Design review of the part built by this model. Coordinates are the model's own, in mm. Round coordinates to 2 decimals unless told otherwise and drop trailing zeros. Loops run counter-clockwise (first coordinate to the right, second up) from the corner with the lowest first, then second, coordinate; pieces in that order, holes last. Notation, with made-up numbers: (46, 80.5) - (68, 80.5) arc R35 cw to (68, 118.5) - close; hole circle Ø3 at (-0.75, 52). An arc over 180 degrees is marked (long way). Return JSON: item names as keys, results as strings. Group by question number.
(1) We need section B-B, the plane x = 0. Write out the cut boundary in (y, z) (3 decimals).
(2) We need section D-D, the plane y = -28. Write out the cut boundary in (x, z).
(3) The part is to be moulded in two halves that separate along Y. For faces 1 (the cylindrical face through (95.38, 30.04, -0.01)), 2 (the cylindrical face through (16.5, -12.3, 0)), 3 (the cylindrical face through (-21.24, 10.87, -0.01)), 4 (the flat face through (21, 1, -0.9)), say which applies: pulls with the +Y half, pulls with the -Y half, needs draft (parallel to the pull), parting line crosses it, or undercut.
(4) We need section C-C, the plane y = 0. Write out the cut boundary in (x, z) (3 decimals).
(5) Clearance check with flat-ended pins moving along their axes: pin 1 (1 mm diameter, centred on x = 70, z = -0.5, fed in from +Y); pin 2 (7 mm diameter, centred on x = 18.62, y = 10.75, fed in from +Z). State where each tip first meets the part, or that it passes through.
(6) Wall thickness on L1, parallel to Y at x = 0, z = 0.25 (3 decimals); L2, parallel to X at y = -23, z = 0.5; L3, parallel to Y at x = 6, z = -0.1: over which ranges is each line inside the solid? List them lowest first. Write a range as [from, to].
(7) We need section A-A, the plane z = 0.55. Write out the cut boundary in (x, y) (3 decimals), and give its area (3 significant figures).
from build123d import *

# Parameters (mm, degrees)
BOSS_EXTRUDE1_DEPTH      = 0.9
BOSS_EXTRUDE1_DEPTH_BACK = 0.9
SKETCH1_R                = 100
SKETCH1_R_2              = 16.625
SKETCH1_R_3              = 2.625


with BuildPart() as part:
    # Sketch1 → Boss-Extrude1 (new, two sides: drawn at the far end of the back side and taken through both)
    with BuildSketch(Plane.XY.offset(-BOSS_EXTRUDE1_DEPTH_BACK)):
        Circle(SKETCH1_R)
        Circle(SKETCH1_R_2, mode=Mode.SUBTRACT)
        with Locations((0, 21.5)):
            Circle(SKETCH1_R_3, mode=Mode.SUBTRACT)
        with Locations((18.619546181, 10.75)):
            Circle(SKETCH1_R_3, mode=Mode.SUBTRACT)
        with Locations((18.619546181, -10.75)):
            Circle(SKETCH1_R_3, mode=Mode.SUBTRACT)
        with Locations((0, -21.5)):
            Circle(SKETCH1_R_3, mode=Mode.SUBTRACT)
        with Locations((-18.619546181, -10.75)):
            Circle(SKETCH1_R_3, mode=Mode.SUBTRACT)
        with Locations((-18.619546181, 10.75)):
            Circle(SKETCH1_R_3, mode=Mode.SUBTRACT)
    extrude(amount=BOSS_EXTRUDE1_DEPTH + BOSS_EXTRUDE1_DEPTH_BACK)


solid = part.part
Solutions:
{
 "1": {"outline": "(-100, -0.9) - (-24.125, -0.9) - (-24.125, 0.9) - (-100, 0.9) - close; (-18.875, -0.9) - (-16.625, -0.9) - (-16.625, 0.9) - (-18.875, 0.9) - close; (16.625, -0.9) - (18.875, -0.9) - (18.875, 0.9) - (16.625, 0.9) - close; (24.125, -0.9) - (100, -0.9) - (100, 0.9) - (24.125, 0.9) - close"},
 "2": {"outline": "(-96, -0.9) - (96, -0.9) - (96, 0.9) - (-96, 0.9) - close"},
 "3": {"face 1": "parting line crosses it", "face 2": "undercut", "face 3": "undercut", "face 4": "needs draft"},
 "4": {"outline": "(-100, -0.9) - (-16.625, -0.9) - (-16.625, 0.9) - (-100, 0.9) - close; (16.625, -0.9) - (100, -0.9) - (100, 0.9) - (16.625, 0.9) - close"},
 "5": {"pin 1": "y = 71.9", "pin 2": "z = 0.9"},
 "6": {"L1": "[-100, -24.125], [-18.875, -16.625], [16.625, 18.875], [24.125, 100]", "L2": "[-97.32, -2.15], [2.15, 97.32]", "L3": "[-99.82, -15.5], [15.5, 99.82]"},
 "7": {"outline": "circle Ø200 at (0, 0); hole circle Ø5.25 at (-18.62, -10.75); hole circle Ø5.25 at (-18.62, 10.75); hole circle Ø33.25 at (0, 0); hole circle Ø5.25 at (0, -21.5); hole circle Ø5.25 at (0, 21.5); hole circle Ø5.25 at (18.62, -10.75); hole circle Ø5.25 at (18.62, 10.75)", "area": "30,400 mm^2"}
}
